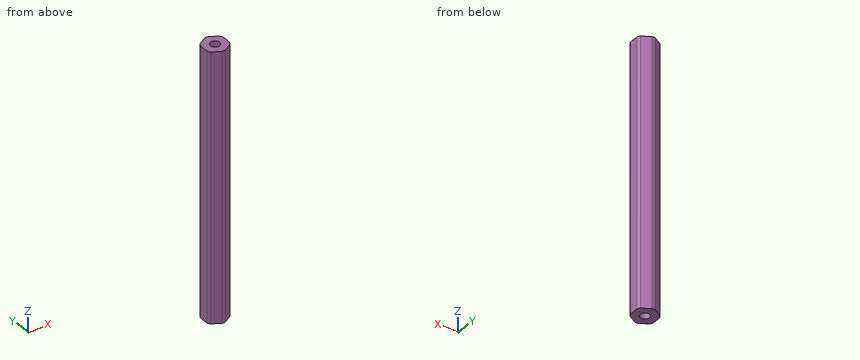
Autodesk Inventor part; units mm, degrees
ref_plane "YZ Plane" through (0, 0, 0) normal (1, 0, 0) x (0, 1, 0)
ref_plane "XZ Plane" through (0, 0, 0) normal (0, 1, 0) x (-1, 0, 0)
ref_plane "XY Plane" through (0, 0, 0) normal (0, 0, 1) x (1, 0, 0)
sketch "Sketch1" plane through (0, 0, 0) normal (0, 0, 1) x (1, 0, 0)
  line L0 (-6.35, -3.6662) -> (-6.35, 3.6662)
  line L1 (-6.35, 3.6662) -> (0, 7.3323)
  line L2 (0, 7.3323) -> (6.35, 3.6662)
  line L3 (6.35, 3.6662) -> (6.35, -3.6662)
  line L4 (6.35, -3.6662) -> (0, -7.3323)
  line L5 (0, -7.3323) -> (-6.35, -3.6662)
  point P0 (0, 0)
  point P1 (0, 0)
  dimension "Size" = 12.7
extrude "Extrusion1" add sketch "Sketch1" along normal mid plane 149.225
sketch "Sketch3" plane through (0, 0, 74.6125) normal (0, 0, 1) x (1, 0, 0)
  line L0 (-6.35, 3.6662) -> (0, 7.3323) construction
  line L1 (0, 7.3323) -> (6.35, 3.6662) construction
  line L2 (6.35, 3.6662) -> (6.35, -3.6662) construction
  line L3 (6.35, -3.6662) -> (0, -7.3323) construction
  line L4 (0, -7.3323) -> (-6.35, -3.6662) construction
  line L5 (-6.35, -3.6662) -> (-6.35, 3.6662) construction
  point P0 (0, 0)
hole "Hole1" at (0, 0, 74.6125) direction (0, 0, -1) diameter 5.1054 end through all
sketch "Sketch4" plane through (0, 0, 74.6125) normal (0, 0, 1) x (1, 0, 0)
  circle A0 centre (0, 0) radius 2.5527 construction
  line L0 (-6.35, 3.6662) -> (0, 7.3323) construction
  line L1 (0, 7.3323) -> (6.35, 3.6662) construction
  line L2 (6.35, 3.6662) -> (6.35, -3.6662) construction
  line L3 (6.35, -3.6662) -> (0, -7.3323) construction
  line L4 (0, -7.3323) -> (-6.35, -3.6662) construction
  line L5 (-6.35, -3.6662) -> (-6.35, 3.6662) construction
  circle A1 centre (0, 0) radius 6.8771
  circle A2 centre (0, 0) radius 8.89
  dimension "thunder" = 13.7541
  dimension "d16" = 17.78
extrude "Extrusion3" cut sketch "Sketch4" against normal through all
equation "\"bearing\" = 25.4"
properties part number "GP3-003" material "Aluminum 6061"
Part model, mm, in its own coordinate system. Give positions to 0.01 mm unless a question says otherwise; leave off trailing zeros. Order: outer loops, then holes, each group sorted by start corner. A loop starts at its lowest first (then second) coordinate and runs counter-clockwise, first axis right, second up. Notation, with made-up numbers: M -40,42.25 L -31,42.25 A22 ccw -31,74.25 Z; hole C 45,7 d5. An arc over 180 degrees is marked long. Use a Markdown table: item, result. Add a question column.
(1) Saw through at B-B, the plane y = 0. Give the cut face in (x, z).
(2) Probe line 1 along Y through (x, z) = (0, 23.5); line 2 along X through (y, z) = (0, -44); line 3 along X through (y, z) = (-2, 14.5). List the from-to ranges inside material, lowest first. Write a range as [from, to].
(3) Saw through at A-A, the plane z = -39. Give the cut face in (x, y), and give its area (3 significant figures).
(4) Drop flat-ended pins along their axis: P1, Ø2, axis at x = -3, z = -37, coming from the +Y side; P2, Ø2, axis at x = -2, z = 47, coming from the +Y side; P3, Ø3, axis at y = 4.5, z = 10.5, coming from the +X side. Give the stop position or say it passes through.
Answer key:
| question | item | result |
|---|---|---|
| 1 | outline | M -6.35,-74.61 L -2.55,-74.61 L -2.55,74.61 L -6.35,74.61 Z; M 2.55,-74.61 L 6.35,-74.61 L 6.35,74.61 L 2.55,74.61 Z |
| 2 | line 1 | [-6.88, -2.55], [2.55, 6.88] |
| 2 | line 2 | [-6.35, -2.55], [2.55, 6.35] |
| 2 | line 3 | [-6.35, -1.59], [1.59, 6.35] |
| 3 | outline | M -6.35,-2.64 A6.88 ccw -5.46,-4.18 L -0.89,-6.82 A6.88 ccw 0.89,-6.82 L 5.46,-4.18 A6.88 ccw 6.35,-2.64 L 6.35,2.64 A6.88 ccw 5.46,4.18 L 0.89,6.82 A6.88 ccw -0.89,6.82 L -5.46,4.18 A6.88 ccw -6.35,2.64 Z; hole C 0,0 d5.11 |
| 3 | area | 117 mm^2 |
| 4 | P1 | y = 6.18 |
| 4 | P2 | y = 6.75 |
| 4 | P3 | x = 6.19 |
